Build history of the part. All positions in model axes, mm. A direction names the side the tool comes from. Give positions to 0.01 mm unless a question says otherwise; leave off trailing zeros. Order: outer loops, then holes, each group sorted by start corner. A loop starts at its lowest first (then second) coordinate and runs counter-clockwise, first axis right, second up. Notation, with made-up numbers: M 78,73 L 92,73 A20 ccw 92,79 Z; hole C -11.75,-15.5 d8. An arc over 180 degrees is marked long. One line per item, written item: value.
from build123d import *

# Parameters (mm, degrees)
BOX_W           = 70
BOX_H           = 42
BOX_DEPTH       = 17
SKETCH_R        = 1.75
POCKET_DEPTH    = 70.001
POCKET001_DEPTH = 50
POCKET002_DEPTH = 35
SKETCH003_R     = 6.75
POCKET003_DEPTH = 17.001
SKETCH004_R     = 8.25
POCKET004_DEPTH = 7.3
SKETCH005_R     = 8.25
POCKET005_DEPTH = 4.2


with BuildPart() as part:
    # Box → Box (new body)
    with BuildSketch(Plane.XY):
        with Locations((35, 21)):
            Rectangle(BOX_W, BOX_H)
    extrude(amount=BOX_DEPTH)

    # Sketch (on Face2 of BaseFeature) → Pocket (cut, through all)
    with BuildSketch(Plane.YZ.offset(70)):
        with Locations((5.5, 13.25)):
            Circle(SKETCH_R)
        with Locations((36.5, 13.25)):
            Circle(SKETCH_R)
    extrude(amount=-POCKET_DEPTH, mode=Mode.SUBTRACT)

    # Sketch001 (on Face2 of BaseFeature) → Pocket001 (cut)
    with BuildSketch(Plane.YZ.offset(70)):
        Polygon((4, 17), (0, 17), (0, 13), align=None)
        Polygon((38, 17), (42, 17), (42, 13), align=None)
    extrude(amount=-POCKET001_DEPTH, mode=Mode.SUBTRACT)

    # Sketch002 (on Face8 of Pocket001) → Pocket002 (cut)
    with BuildSketch(Plane.YZ.offset(70)):
        Polygon((4, 17), (0, 13), (0, 10.5), (3.5, 7), (38.5, 7), (42, 10.5), (42, 13), (38, 17), align=None)
    extrude(amount=-POCKET002_DEPTH, mode=Mode.SUBTRACT)

    # Sketch003 (on Face3 of Pocket002) → Pocket003 (cut, through all)
    with BuildSketch(Plane.XY.offset(17)):
        with Locations((27, 27)):
            Circle(SKETCH003_R)
    extrude(amount=-POCKET003_DEPTH, mode=Mode.SUBTRACT)

    # Sketch004 (on Face3 of Pocket003) → Pocket004 (cut)
    with BuildSketch(Plane.XY.offset(17)):
        with Locations((27, 27)):
            Circle(SKETCH004_R)
    extrude(amount=-POCKET004_DEPTH, mode=Mode.SUBTRACT)

    # Sketch005 (on Face4 of Pocket004) → Pocket005 (cut)
    with BuildSketch(Plane(origin=(0, 0, 0), x_dir=(1, 0, 0), z_dir=(0, 0, -1))):
        with Locations((27, -27)):
            Circle(SKETCH005_R)
    extrude(amount=-POCKET005_DEPTH, mode=Mode.SUBTRACT)


solid = part.part
1) Saw through at D-D, the plane x = 15. Write the cut outline in (y, z).
Check values:
outline: M 0,0 L 42,0 L 42,17 L 0,17 Z; hole C 5.5,13.25 d3.5; hole C 36.5,13.25 d3.5
2) Tool access for faces 1 (the face through (28, 40, 15)), 2 (the face through (28, 2, 15)), 3 (the face through (35, 21, 12)), 4 (the face through (20, 27, 4.2)), 5 (the face through (70, 21, 4)): list every direction of +Z, -Z, +X, -X, +Y, -Y with a clear straight run to the whole face (end or side of a thin tool).
Check values:
face 1: +Z, +X, +Y
face 2: +Z, +X, -Y
face 3: +Z, +X
face 4: -Z
face 5: +Z, -Z, +X, +Y, -Y
3) Saw through at B-B, the plane y = 5.5. Write the cut outline in (x, z).
Check values:
outline: M 0,0 L 70,0 L 70,7 L 35,7 L 35,11.5 L 0,11.5 Z; M 0,15 L 35,15 L 35,17 L 0,17 Z
4) Saw through at A-A, the plane x = 26. Write the cut outline in (y, z), then the cut area to 3 significant figures.
Check values:
outline: M 0,0 L 18.81,0 L 18.81,4.2 L 20.32,4.2 L 20.32,9.7 L 18.81,9.7 L 18.81,17 L 4,17 L 0,13 Z; M 33.68,4.2 L 35.19,4.2 L 35.19,0 L 42,0 L 42,13 L 38,17 L 35.19,17 L 35.19,14.41 A1.75 cw long 35.19,12.09 L 35.19,9.7 L 33.68,9.7 Z; hole C 5.5,13.25 d3.5
area: 418 mm^2
5) Saw through at C-C, the plane z = 6.25. Write the cut outline in (x, y).
Check values:
outline: M 0,0 L 70,0 L 70,42 L 0,42 Z; hole C 27,27 d13.5
6) Mould opens along X. For faces 6 (the face through (20, 40.5, 15.5)), 7 (the face through (18.757, 27.334, 13.401)), 8 (the face through (53, 21, 7)) say: released by +X, released by -X, zero draft, split by the parting line, or undercut.
Check values:
face 6: released by +X
face 7: undercut
face 8: zero draft
7) Drill centre lines: probe 1 along Y at (x, z) = (27, 2.65); probe 2 along Y at (x, z) = (27, 5.5); probe 3 along Y at (x, z) = (27, 12.5). Where is each one in solid material? Low to high. Write a range as from..to.
Check values:
probe 1: 0..18.75, 35.25..42
probe 2: 0..20.25, 33.75..42
probe 3: 0..3.92, 7.08..18.75, 38.08..42
8) Pin check, flat tips, straight feed: pin 1 (6 mm diameter, centred on y = 15.5, z = 11, fed in from +X); pin 2 (17.5 mm diameter, centred on x = 57, y = 16, fed in from +Z); pin 3 (6 mm diameter, centred on x = 18.5, z = 2.5, fed in from -Y). Stop position of each tip, or through.
Check values:
pin 1: x = 35
pin 2: z = 7
pin 3: y = 0
